Build history of the part. All positions in model axes, mm. A direction names the side the tool comes from. Give positions to 0.01 mm unless a question says otherwise; leave off trailing zeros. Write each loop counter-clockwise with the first axis right and the second up, starting at its lowest first coordinate (ties: lowest second). Pieces come first, ordered by that corner, then holes. Notation, with made-up numbers: (55.5, 9.5) - (99.5, 9.5) arc R15 cw to (99.5, 31.5) - close; hole circle Ø4 at (57, 76.5). An arc over 180 degrees is marked (long way). Use one line per item in the form item = value. Start each with the question number.
Autodesk Inventor part; units mm, degrees
ref_plane "YZ Plane" through (0, 0, 0) normal (1, 0, 0) x (0, 1, 0)
ref_plane "XZ Plane" through (0, 0, 0) normal (0, 1, 0) x (-1, 0, 0)
ref_plane "XY Plane" through (0, 0, 0) normal (0, 0, 1) x (1, 0, 0)
sketch "Esquisse1" plane through (0, 0, 0) normal (0, 1, 0) x (-1, 0, 0)
  circle A0 centre (0, 0) radius 9.5
  circle A1 centre (0, 0) radius 2.05 construction
  line L0 (0, 9.5) -> (0, -9.5) construction
  line L1 (-9.5, 0) -> (9.5, 0) construction
  circle A2 centre (0, -6) radius 2.05
  circle A3 centre (0, 6) radius 2.05
  circle A4 centre (0, 0) radius 2.05 construction
  circle A5 centre (6, 0) radius 2.05
  circle A6 centre (-6, 0) radius 2.05
  circle A7 centre (0, 0) radius 2.05 construction
  dimension "d0" = 19
  dimension "d1" = 4.1
  dimension "d4" = 6
  dimension "d7" = 6
  dimension "d12" = 6
  dimension "d15" = 6
extrude "Extrusion1" add sketch "Esquisse1" along normal blind 3
sketch "Esquisse2" plane through (0, 3, 0) normal (0, 1, 0) x (1, 0, 0)
  circle A0 centre (0, 0) radius 9.5 construction
  circle A1 centre (0, 0) radius 1.5
  dimension "d20" = 3
extrude "Extrusion2" cut sketch "Esquisse2" against normal through all
sketch "Sketch3" plane through (0, 0, 0) normal (0, -1, 0) x (1, 0, 0)
  circle A0 centre (-6, 0) radius 2.05
  circle A1 centre (0, 6) radius 2.05
  circle A2 centre (6, 0) radius 2.05
  circle A3 centre (0, -6) radius 2.05
  circle A4 centre (0, -6) radius 2.55
  circle A5 centre (6, 0) radius 2.55
  circle A6 centre (-6, 0) radius 2.55
  circle A7 centre (0, 6) radius 2.55
  point P0 (0, 0)
  dimension "d23" = 5.1
  dimension "d24" = 5.1
  dimension "d25" = 5.1
  dimension "d26" = 5.1
extrude "Extrusion3" cut sketch "Sketch3" against normal blind 1
sketch "Sketch4" plane through (0, 3, 0) normal (0, 1, 0) x (1, 0, 0)
  circle A0 centre (0, -6) radius 2.55
  circle A1 centre (0, -6) radius 2.55
  circle A2 centre (-6, 0) radius 2.55
  circle A3 centre (-6, 0) radius 2.55
  circle A4 centre (0, 6) radius 2.55
  circle A5 centre (0, 6) radius 2.55
  circle A6 centre (6, 0) radius 2.55
  circle A7 centre (6, 0) radius 2.55
  point P0 (0, 0)
extrude "Extrusion4" cut sketch "Sketch4" against normal blind 1
properties part number "XL320_HubToOllo"
(1) Cut at C-C, the plane x = -6.25. Give the cut face in (y, z).
(2) Wall check: line 1 (Z direction, x = 0, y = 2.75); line 2 (Z direction, x = -1.25, y = 2.6); line 3 (X direction, y = 1.2, z = -1.25). Give the ranges that are in metal, low to high. Write a range as from..to.
(3) Cut at A-A, the plane x = 0. State how many separate pieces and enclosed holes the cut face has, then the cut area to 3 significant figures.
(4) Pin check, flat tips, straight feed: pin 1 Ø4.5 at (x, z) = (0, 6) entering from -Y; pin 2 Ø4.5 at (x, z) = (-6, 0) entering from +Y; pin 3 Ø1.5 at (y, z) = (1, -7) entering from +X; pin 4 Ø3 at (x, z) = (-6, 0) entering from +Y. Stop position of each tip, or through.
(5) Which spindle directions (+Z, -Z, +X, -X, +Y, -Y) get a long thin tool onto all of the face, cutting with end or side? Do faces 4 (the cylindrical face through (8.43, 0.49, 0.77)), 5 (the flat face through (-2, 2, 5)), 6 (the cylindrical face through (8.05, 1.49, -0.09)). Say none if no direction does.
(6) Cut at D-D, the plane y = 1.4. Give the cut face in (x, z).
(7) Two-plate mould, pull along Z, no slides. Class faces 1 (the flat face through (-2, 2, -7)), 2 (the flat face through (0, 0, -2)), 3 (the cylindrical face through (-4.38, 1.48, 8.43)): +Z half, -Z half, draft (parallel to the pull), parting line (faces both ways), or undercut.
Solution:
q1.outline = (0, -7.15) - (3, -7.15) - (3, -2.54) - (2, -2.54) - (2, -2.03) - (1, -2.03) - (1, -2.54) - (0, -2.54) - close; (0, 2.54) - (1, 2.54) - (1, 2.03) - (2, 2.03) - (2, 2.54) - (3, 2.54) - (3, 7.15) - (0, 7.15) - close
q2.line_1 = -9.5..-8.55, -3.45..-1.5, 1.5..3.45, 8.55..9.5
q2.line_2 = -9.42..-8.22, -3.78..-0.83, 0.83..3.78, 8.22..9.42
q2.line_3 = -9.42..-7.62, -4.38..-0.83, 0.83..4.38, 7.62..9.42
q3.separate_pieces = 4
q3.enclosed_holes = 0
q3.area = 19.4 mm2
q4.pin_1 = 1
q4.pin_2 = 2
q4.pin_3 = 7.15
q4.pin_4 = through
q5.face_4 = -Y
q5.face_5 = +Y
q5.face_6 = +Y, -Y
q6.outline = circle Ø19 at (0, 0); hole circle Ø4.1 at (-6, 0); hole circle Ø4.1 at (0, -6); hole circle Ø4.1 at (0, 6); hole circle Ø3 at (0, 0); hole circle Ø4.1 at (6, 0)
q7.face_1 = undercut
q7.face_2 = draft
q7.face_3 = parting line
